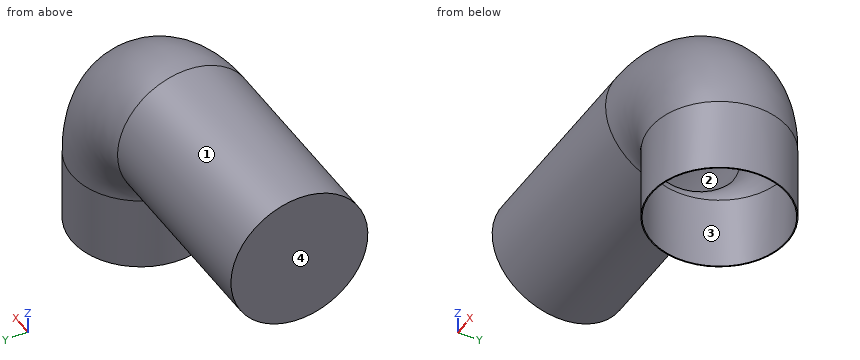
```python
from build123d import *

# Parameters (mm, degrees)
SWEEP1_PROFILE_R = 34
SHELL1_T         = -0.5


with BuildPart() as part:
    # Sweep1: sweep along a curve in space
    with BuildLine() as sweep1_path:
        Line((0, 0, 0), (0, 0, 36.87))
        ThreePointArc((0, 0, 36.87), (-11.715728753, 0, 65.154271247), (-40, 0, 76.87))
        Line((-40, 0, 76.87), (-140, 0, 76.87))
    # Sweep1 profile (on start of the path) → Sweep1 (sweep)
    with BuildSketch(Plane.XY):
        Circle(SWEEP1_PROFILE_R)
    sweep(path=sweep1_path.line)

    # Shell1
    shell1_openings = [part.faces().sort_by_distance(p)[0] for p in [
        (0, 0, 0),
    ]]
    offset(amount=SHELL1_T, openings=shell1_openings, kind=Kind.INTERSECTION)


solid = part.part
```
Design review of the part built by this model. Coordinates are the model's own, in mm. Face numbers are marked on the shaded views. Give positions to 0.01 mm unless a question says otherwise; leave off trailing zeros. Order: outer loops, then holes, each group sorted by start corner. A loop starts at its lowest first (then second) coordinate and runs counter-clockwise, first axis right, second up. Notation, with made-up numbers: (83.5, -35) -> (142.5, -35) arc R19 cw to (142.5, -4) -> close; hole circle Ø9 at (29, 71). An arc over 180 degrees is marked (long way). Write item = value, one per line. Start each with the question number.
(1) To check wall thickness, follow line 1 along Y through (x, z) = (-114, 76.87); line 2 along Z through (x, y) = (-101, 0); line 3 along Z through (x, y) = (-54, 1.5). State the ranges of each line that lie inside material, in increasing order.
(2) Mouldability with a two-part tool opening along X and no side actions: class the marked faces 1, 2, 3 and 4 as +X half, -X half, draft (parallel to the pull), parting line (faces both ways), or undercut.
(3) We need section A-A on y = 0. Write out the cut boundary in (x, z).
(4) We need section D-D on y = -21.5. Write out the cut boundary in (x, z), plus the area to 3 significant figures.
(5) We need section B-B on z = 8. Write out the cut boundary in (x, y).
(6) We need section C-C on x = -76. Write out the cut boundary in (y, z), plus the area to 3 significant figures.
(7) For pin 1 (20 mm diameter, centred on y = -14, z = 63.5, fed in from +X); pin 2 (4 mm diameter, centred on x = -75, y = 21, fed in from -Z); pin 3 (10 mm diameter, centred on x = -23.5, y = 15.5, fed in from +Z), all flat-tipped, find the tip position at first contact; note any pin that passes through.
Numbers:
q1.line_1 = -34 to -33.5, 33.5 to 34
q1.line_2 = 42.87 to 43.37, 110.37 to 110.87
q1.line_3 = 42.9 to 43.4, 110.34 to 110.84
q2.face_1 = draft
q2.face_2 = undercut
q2.face_3 = undercut
q2.face_4 = -X half
q3.outline = (-140, 42.87) -> (-40, 42.87) arc R6 cw to (-34, 36.87) -> (-34, 0) -> (-33.5, 0) -> (-33.5, 36.87) arc R6.5 ccw to (-40, 43.37) -> (-139.5, 43.37) -> (-139.5, 110.37) -> (-40, 110.37) arc R73.5 cw to (33.5, 36.87) -> (33.5, 0) -> (34, 0) -> (34, 36.87) arc R74 ccw to (-40, 110.87) -> (-140, 110.87) -> close
q4.outline = (-140, 50.53) -> (-40, 50.53) arc R13.66 cw to (-26.34, 36.87) -> (-26.34, 0) -> (-25.69, 0) -> (-25.69, 36.87) arc R14.31 ccw to (-40, 51.18) -> (-139.5, 51.18) -> (-139.5, 102.56) -> (-40, 102.56) arc R65.69 cw to (25.69, 36.87) -> (25.69, 0) -> (26.34, 0) -> (26.34, 36.87) arc R66.34 ccw to (-40, 103.21) -> (-140, 103.21) -> close
q4.area = 285 mm^2
q5.outline = circle Ø68 at (0, 0); hole circle Ø67 at (0, 0)
q6.outline = circle Ø68 at (0, 76.87); hole circle Ø67 at (0, 76.87)
q6.area = 106 mm^2
q7.pin_1 = 30.64
q7.pin_2 = 48.67
q7.pin_3 = 107.61
